from build123d import *

# Parameters (mm, degrees)
SKETCH1_W           = 26
SKETCH1_H           = 10
BOSS_EXTRUDE1_DEPTH = 20
CUT_EXTRUDE1_DEPTH  = 21
SKETCH3_R           = 1.5
CUT_EXTRUDE2_DEPTH  = 10


with BuildPart() as part:
    # Sketch1 → Boss-Extrude1 (new body)
    with BuildSketch(Plane(origin=(0, 0, 0), x_dir=(1, 0, 0), z_dir=(0, 1, 0))):
        with Locations((13, 5)):
            Rectangle(SKETCH1_W, SKETCH1_H)
    extrude(amount=BOSS_EXTRUDE1_DEPTH)

    # Sketch2 → Cut-Extrude1 (cut, through all)
    with BuildSketch(Plane(origin=(0, 20, 0), x_dir=(1, 0, 0), z_dir=(0, 1, 0))):
        with BuildLine():
            Line((6.5, 0), (19.5, 0))
            ThreePointArc((19.5, 0), (13, 6.5), (6.5, 0))
        make_face()
    extrude(amount=-CUT_EXTRUDE1_DEPTH, mode=Mode.SUBTRACT)

    # Sketch3 → Cut-Extrude2 (cut)
    with BuildSketch(Plane(origin=(0, 0, -10), x_dir=(-1, 0, 0), z_dir=(0, 0, -1))):
        with Locations((-23, 17)):
            Circle(SKETCH3_R)
        with Locations((-3, 17)):
            Circle(SKETCH3_R)
        with Locations((-3, 3)):
            Circle(SKETCH3_R)
        with Locations((-23, 3)):
            Circle(SKETCH3_R)
    extrude(amount=-CUT_EXTRUDE2_DEPTH, mode=Mode.SUBTRACT)


solid = part.part
Model file for the job. Use its own axes, mm. Give positions to 0.01 mm unless a question says otherwise; leave off trailing zeros. Loops run counter-clockwise (first coordinate to the right, second up) from the corner with the lowest first, then second, coordinate; pieces in that order, holes last.
1) Saw through at B-B (y = 3). Write the cut outline in (x, z).
2) Saw through at D-D (z = -7). Write the cut outline in (x, y).
3) Wall check: line 1 (Y direction, x = 3, z = -4); line 2 (X direction, y = 1.25, z = -0.25); line 3 (Y direction, x = 1.75, z = -2). Give the ranges that are in metal, low to high.
4) Pull direction X, two halves, no side cores. Call faces 1 (the flat face through (0, 10, -5)), 2 (the cylindrical face through (3.195, 18.487, -5.07)), 3 (the flat face through (23, 10, 0)): +X half, -X half, draft (parallel to the pull), parting line (faces both ways), or undercut.
5) Saw through at C-C (x = 23). Write the cut outline in (y, z), plus the area to 3 significant figures.
6) Saw through at A-A (z = -2.5). Write the cut outline in (x, y), plus the area to 3 significant figures.
7) Flat gauge pin, fed straight in: pin 1 Ø3 at (x, z) = (18.5, -6.5) entering from -Y. Where does the tip first touch, or does it go through?
Answer block:
1. outline: (0, -10) - (1.5, -10) - (1.5, 0) - (0, 0) - close; (4.5, -10) - (21.5, -10) - (21.5, 0) - (19.5, 0) arc R6.5 cw to (6.5, 0) - (4.5, 0) - close; (24.5, -10) - (26, -10) - (26, 0) - (24.5, 0) - close
2. outline: (0, 0) - (26, 0) - (26, 20) - (0, 20) - close; hole circle Ø3 at (3, 3); hole circle Ø3 at (3, 17); hole circle Ø3 at (23, 3); hole circle Ø3 at (23, 17)
3. line 1: y = 0 to 1.5, 4.5 to 15.5, 18.5 to 20
3. line 2: x = 0 to 6.5, 19.5 to 26
3. line 3: y = 0 to 2.17, 3.83 to 16.17, 17.83 to 20
4. face 1: -X half
4. face 2: undercut
4. face 3: draft
5. outline: (0, -10) - (1.5, -10) - (1.5, 0) - (0, 0) - close; (4.5, -10) - (15.5, -10) - (15.5, 0) - (4.5, 0) - close; (18.5, -10) - (20, -10) - (20, 0) - (18.5, 0) - close
5. area: 140 mm2
6. outline: (0, 0) - (7, 0) - (7, 20) - (0, 20) - close; (19, 0) - (26, 0) - (26, 20) - (19, 20) - close; hole circle Ø3 at (3, 3); hole circle Ø3 at (3, 17); hole circle Ø3 at (23, 3); hole circle Ø3 at (23, 17)
6. area: 252 mm2
7. pin 1: stops at y = 0
